Build history of the part. All positions in model axes, mm. A direction names the side the tool comes from. Give positions to 0.01 mm unless a question says otherwise; leave off trailing zeros. Write each loop counter-clockwise with the first axis right and the second up, starting at its lowest first coordinate (ties: lowest second). Pieces come first, ordered by that corner, then holes. Notation, with made-up numbers: (14, -32.5) - (31, -32.5) arc R23 cw to (31, 0.5) - close; hole circle Ø7 at (-1, 61). An arc over 180 degrees is marked (long way). Use one line per item in the form item = value. Start each with the question number.
from build123d import *

# Parameters (mm, degrees)
SKETCH_1_W                  = 203
SKETCH_1_H                  = 35
EXTRUDE_1_DEPTH             = 5
HOLE_WIZARD_M5_1_AT_2_COUNT = 2
HOLE_WIZARD_M5_1_AT_2_PITCH = 20
SKETCH_4_W                  = 40
SKETCH_4_H                  = 15
CUT_EXTRUDE_1_DEPTH         = 10
FILLET_1_R                  = 5
HOLE_WIZARD_4_2_4_2_1_D     = 4.2
FILLET_1_OF_MIRROR_2_R      = 5


with BuildPart() as part:
    # 草图1 → 凸台-拉伸1 (new body, symmetric)
    with BuildSketch(Plane.XY):
        Rectangle(SKETCH_1_W, SKETCH_1_H)
    extrude(amount=EXTRUDE_1_DEPTH, both=True)

    # 草图2 → M5 螺纹孔1 (revolve, cut)
    with BuildSketch(Plane(origin=(-101.5, 10, 0), x_dir=(0, 0, 1), z_dir=(0, 1, 0))):
        Polygon((0, 0), (0, 15.2618073), (2.1, 14), (2.1, 0), align=None)
    hole_wizard_m5_1 = revolve(axis=Axis((-107.85, 10, 0), (1, 0, 0)), mode=Mode.SUBTRACT)

    # M5 螺纹孔1 at 2: M5 螺纹孔1 ×2
    with Locations(*[(0, -i * HOLE_WIZARD_M5_1_AT_2_PITCH, 0) for i in range(1, HOLE_WIZARD_M5_1_AT_2_COUNT)]):
        add(hole_wizard_m5_1, mode=Mode.SUBTRACT)

    # 镜向1: M5 螺纹孔1 across plane
    add(hole_wizard_m5_1.mirror(Plane(origin=(0, 0, 0), x_dir=(0, 0, 1), z_dir=(1, 0, 0))), mode=Mode.SUBTRACT)

    # 镜向1 copy 1 sketch → 镜向1 copy 1 (revolve, cut)
    with BuildSketch(Plane(origin=(101.5, -10, 0), x_dir=(0, 0, 1), z_dir=(0, 1, 0))):
        Polygon((0, 0), (0, -15.2618073), (2.1, -14), (2.1, 0), align=None)
    revolve(axis=Axis((107.85, -10, 0), (1, 0, 0)), mode=Mode.SUBTRACT)

    # 草图4 → 切除-拉伸1 (cut)
    with BuildSketch(Plane(origin=(0, 0, -5), x_dir=(-1, 0, 0), z_dir=(0, 0, -1))):
        with Locations((56.5, 0)):
            Rectangle(SKETCH_4_W, SKETCH_4_H)
    cut_extrude_1 = extrude(amount=-CUT_EXTRUDE_1_DEPTH, mode=Mode.SUBTRACT)

    # 圆角1
    fillet_1_edges = [part.edges().sort_by_distance(p)[0] for p in [
        (-76.5, 7.5, 0),
        (-76.5, -7.5, 0),
        (-36.5, -7.5, 0),
        (-36.5, 7.5, 0),
    ]]
    fillet(fillet_1_edges, radius=FILLET_1_R)

    # Ø4.2 (4.2) 直径孔1 (through all)
    with Locations(Plane(origin=(0, 0, -5), x_dir=(-1, 0, 0), z_dir=(0, 0, -1))):
        with Locations((81.5, 0), (31.5, 0)):
            hole_wizard_4_2_4_2_1 = Hole(HOLE_WIZARD_4_2_4_2_1_D / 2)

    # 镜向2: 切除-拉伸1, Ø4.2 (4.2) 直径孔1 across plane
    add(cut_extrude_1.mirror(Plane(origin=(0, 0, 0), x_dir=(0, 0, 1), z_dir=(1, 0, 0))), mode=Mode.SUBTRACT)
    add(hole_wizard_4_2_4_2_1.mirror(Plane(origin=(0, 0, 0), x_dir=(0, 0, 1), z_dir=(1, 0, 0))), mode=Mode.SUBTRACT)

    # 圆角1 of 镜向2
    fillet_1_of_mirror_2_edges = [part.edges().sort_by_distance(p)[0] for p in [
        (76.5, 7.5, 0),
        (76.5, -7.5, 0),
        (36.5, -7.5, 0),
        (36.5, 7.5, 0),
    ]]
    fillet(fillet_1_of_mirror_2_edges, radius=FILLET_1_OF_MIRROR_2_R)


solid = part.part
(1) Cut at B-B, the plane x = -31.5. Give the cut face in (y, z).
(2) Cut at C-C, the plane x = -73.5. Give the cut face in (y, z).
(3) Two-plate mould, pull along X, no slides. Class faces 4 (the conical face through (-86.46, -10.31, 0.2)), 5 (the cylindrical face through (-33.6, 0.09, 0.07)), 6 (the cylindrical face through (94.598, 7.918, -0.273)): +X half, -X half, draft (parallel to the pull), parting line (faces both ways), or undercut.
(4) Cut at A-A, the plane y = 0. Give the cut face in (x, z).
(5) Pin check, flat tips, straight feed: pin 1 Ø2.5 at (y, z) = (-10, 0) entering from +X; pin 2 Ø5.5 at (x, y) = (-81.5, 0) entering from +Z; pin 3 Ø4 at (x, y) = (31.5, 0) entering from +Z. Stop position of each tip, or through.
(6) Wall check: line 1 (Y direction, x = 96, z = 0); line 2 (Y direction, x = -48.5, z = -4); line 3 (Y direction, x = 31.5, z = 0.5). Give the ranges that are in metal, low to high. Write a range as from..to.
(7) Which spindle directions (+Z, -Z, +X, -X, +Y, -Y) get a long thin tool onto all of the face, cutting with end or side? Do faces 1 (the conical face through (86.46, -10.31, 0.2)), 2 (the flat face through (36.5, 0, 0)), 3 (the cylindrical face through (-94.598, 7.918, -0.273)). Say none if no direction does.
Solution:
q1.outline = (-17.5, -5) - (-2.1, -5) - (-2.1, 5) - (-17.5, 5) - close; (2.1, -5) - (17.5, -5) - (17.5, 5) - (2.1, 5) - close
q2.outline = (-17.5, -5) - (-7.08, -5) - (-7.08, 5) - (-17.5, 5) - close; (7.08, -5) - (17.5, -5) - (17.5, 5) - (7.08, 5) - close
q3.face_4 = -X half
q3.face_5 = undercut
q3.face_6 = draft
q4.outline = (-101.5, -5) - (-83.6, -5) - (-83.6, 5) - (-101.5, 5) - close; (-79.4, -5) - (-76.5, -5) - (-76.5, 5) - (-79.4, 5) - close; (-36.5, -5) - (-33.6, -5) - (-33.6, 5) - (-36.5, 5) - close; (-29.4, -5) - (29.4, -5) - (29.4, 5) - (-29.4, 5) - close; (33.6, -5) - (36.5, -5) - (36.5, 5) - (33.6, 5) - close; (76.5, -5) - (79.4, -5) - (79.4, 5) - (76.5, 5) - close; (83.6, -5) - (101.5, -5) - (101.5, 5) - (83.6, 5) - close
q5.pin_1 = 86.99
q5.pin_2 = 5
q5.pin_3 = through
q6.line_1 = -17.5..-12.1, -7.9..7.9, 12.1..17.5
q6.line_2 = -17.5..-7.5, 7.5..17.5
q6.line_3 = -17.5..-2.1, 2.1..17.5
q7.face_1 = +X
q7.face_2 = +Z, -Z
q7.face_3 = -X
